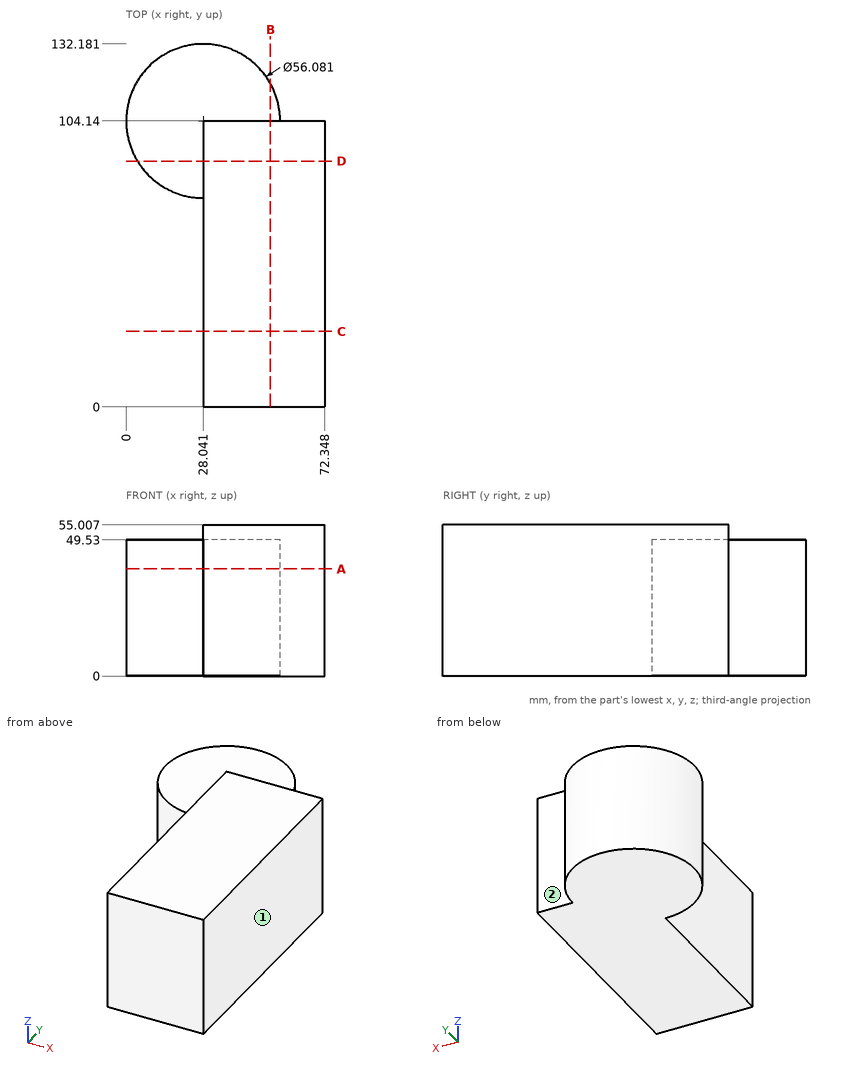
Source: three-view drawing plus pictorial views. Frame: mm from the lowest corner of the part. A direction names the side the tool comes from. Round coordinates to 2 decimals unless told otherwise and drop trailing zeros. Order: outer loops, then holes, each group sorted by start corner. A loop starts at its lowest first (then second) coordinate and runs counter-clockwise, first axis right, second up. Notation, with made-up numbers: (27.5, 57.25) - (33.5, 57.25) arc R17 ccw to (33.5, 82.25) - close; hole circle Ø2 at (4, 2.25). An arc over 180 degrees is marked (long way). Answer in a Markdown table with one row per item.
Item 1: Section query C-C (y = 27.5). Return the cut outline in (x, z).
Model answer:
| item | result |
|---|---|
| outline | (28.04, 0) - (72.35, 0) - (72.35, 55.01) - (28.04, 55.01) - close |
Item 2: Reachability of the marked faces 1 and 2 from +Z, -Z, +X, -X, +Y, -Y: full face, straight path, thin tool, end or side. Return the list, or none.
Model answer:
| item | result |
|---|---|
| face 1 | +Z, -Z, +X, +Y, -Y |
| face 2 | +Z, +X, +Y |
Item 3: Pin query (flat end, axial travel): pin 1 (16.5 mm diameter, centred on y = 34, z = 37.5, fed in from -X); pin 2 (4 mm diameter, centred on x = 43.5, z = 46, fed in from -Y); pin 3 (1.5 mm diameter, centred on x = 43.5, z = 44.5, fed in from +Y); pin 4 (8 mm diameter, centred on x = 48, z = 29, fed in from +Y) (1 decimal). Return the tip coordinate at first contact, or that it passes through.
Model answer:
| item | result |
|---|---|
| pin 1 | stops at x = 28.04 |
| pin 2 | stops at y = 0 |
| pin 3 | stops at y = 128.01 |
| pin 4 | stops at y = 127.2 |
Item 4: Line query: line 1 (Y direction, x = 47, z = 52.5); line 2 (Z direction, x = 25.5, y = 100.5); line 3 (X direction, y = 44, z = 37.5). Output: solid intervals per line, ascending.
Model answer:
| item | result |
|---|---|
| line 1 | y = 0 to 104.14 |
| line 2 | z = 0 to 49.53 |
| line 3 | x = 28.04 to 72.35 |
Item 5: Section query A-A (z = 39). Return the cut outline in (x, y).
Model answer:
| item | result |
|---|---|
| outline | (28.04, 0) - (72.35, 0) - (72.35, 104.14) - (56.08, 104.14) arc R28.04 ccw (long way) to (28.04, 76.1) - close |
Item 6: Section query B-B (x = 52.5). Return the cut outline in (y, z).
Model answer:
| item | result |
|---|---|
| outline | (0, 0) - (117.85, 0) - (117.85, 49.53) - (104.14, 49.53) - (104.14, 55.01) - (0, 55.01) - close |
Item 7: Section query D-D (y = 89.5). Return the cut outline in (x, z) (1 decimal), then the cut area to 3 significant figures.
Model answer:
| item | result |
|---|---|
| outline | (4.1, 0) - (72.3, 0) - (72.3, 55) - (28, 55) - (28, 49.5) - (4.1, 49.5) - close |
| area | 3,620 mm² |
